Can you work these out from the drawing? Everything is in mm from the part's minimum corner. Give positions to 0.01 mm unless a question says otherwise; leave off trailing zeros. Loops run counter-clockwise (first coordinate to the right, second up) from the corner with the lowest first, then second, coordinate; pieces in that order, holes last. Notation, with made-up numbers: (25, 13.5) -> (50, 13.5) arc R23 ccw to (50, 36.5) -> close; hole circle Ø10 at (47.5, 67). An arc over 180 degrees is marked (long way). Return JSON: item names as keys, results as strings. Group by question number.
Q1. Suppose I cut it at A-A, the plane z = 10. Please give me the cut outline in (x, y).
Q2. I need wall thicknesses on line 1 along X through (y, z) = (2, 10); line 2 along X through (y, z) = (1.4, 20); line 3 along Z through (x, y) = (18, 0.35). Which ranges of each line are inside material? Lowest first, please. Write a range as [from, to].
Q3. Suppose I cut it at C-C, the plane y = 1.85. Count the separate pieces of the cut face and the enclosed holes in it, and give its area (3 significant figures).
Q4. Suppose I cut it at D-D, the plane z = 20. Please give me the cut outline in (x, y), and give its area (4 significant figures).
Q5. Suppose I cut it at B-B, the plane x = 93. Please give me the cut outline in (y, z), and give its area (3 significant figures).
Q6. Will these pins go through, and if not, where does the flat tip stop? pin 1 (1.5 mm diameter, centred on x = 110, y = 1, fed in from +Z); pin 2 (0.9 mm diameter, centred on y = 1, z = 23, fed in from +X).
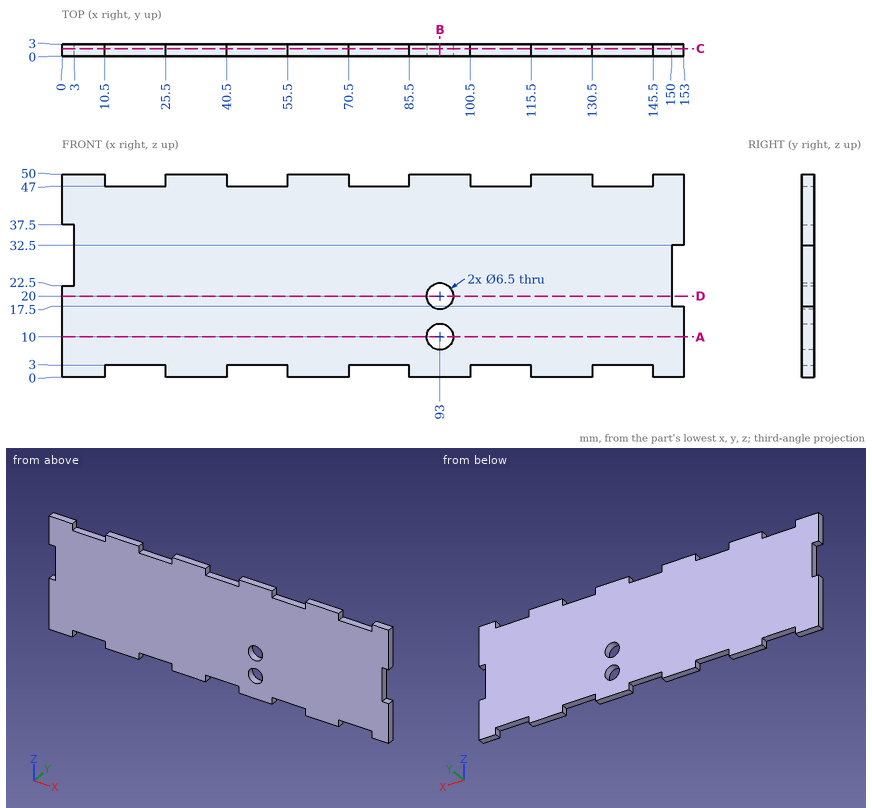
Ans:
{
 "1": {"outline": "(0, 0) -> (89.75, 0) -> (89.75, 3) -> (0, 3) -> close; (96.25, 0) -> (153, 0) -> (153, 3) -> (96.25, 3) -> close"},
 "2": {"line 1": "x = [0, 89.75], [96.25, 153]", "line 2": "x = [0, 89.75], [96.25, 150]", "line 3": "z = [3, 47]"},
 "3": {"separate pieces": "1", "enclosed holes": "2", "area": "7,040 mm^2"},
 "4": {"outline": "(0, 0) -> (89.75, 0) -> (89.75, 3) -> (0, 3) -> close; (96.25, 0) -> (150, 0) -> (150, 3) -> (96.25, 3) -> close", "area": "430.5 mm^2"},
 "5": {"outline": "(0, 0) -> (3, 0) -> (3, 6.75) -> (0, 6.75) -> close; (0, 13.25) -> (3, 13.25) -> (3, 16.75) -> (0, 16.75) -> close; (0, 23.25) -> (3, 23.25) -> (3, 50) -> (0, 50) -> close", "area": "111 mm^2"},
 "6": {"pin 1": "stops at z = 47", "pin 2": "stops at x = 150"}
}
